```python
from build123d import *

# Parameters (mm, degrees)
BOSS_EXTRU_1_DEPTH      = 10
COQUE1_T                = 2
CONG_1_R                = 4
ENL_V_MAT_EXTRU_1_DEPTH = 10


with BuildPart() as part:
    # Esquisse1 → Boss.-Extru.1 (new body)
    with BuildSketch(Plane.XY):
        with BuildLine():
            Line((-33.546223224, -67.598576794), (32.573776776, -67.598576794))
            ThreePointArc((32.573776776, -67.598576794), (34.341543729, -66.866343747), (35.073776776, -65.098576794))
            Line((35.073776776, -65.098576794), (35.073776776, 67.061423206))
            ThreePointArc((35.073776776, 67.061423206), (34.341543729, 68.829190159), (32.573776776, 69.561423206))
            Line((32.573776776, 69.561423206), (-33.546223224, 69.561423206))
            ThreePointArc((-33.546223224, 69.561423206), (-35.313990177, 68.829190159), (-36.046223224, 67.061423206))
            Line((-36.046223224, 67.061423206), (-36.046223224, -65.098576794))
            ThreePointArc((-36.046223224, -65.098576794), (-35.313990177, -66.866343747), (-33.546223224, -67.598576794))
        make_face()
    extrude(amount=BOSS_EXTRU_1_DEPTH)

    # Coque1
    coque1_openings = [part.faces().sort_by_distance(p)[0] for p in [
        (-0.486223224, 0.981423206, 10),
    ]]
    offset(amount=COQUE1_T, openings=coque1_openings, kind=Kind.INTERSECTION)

    # Congé1
    # the kernel refuses this fillet: 4 mm, written as the material it takes off along each edge
    with BuildSketch(Plane(origin=(32.573776776, 71.561423206, -2), x_dir=(0, 0, 1), z_dir=(-1, 0, 0)), Plane(origin=(-33.546223224, -69.598576794, -2), x_dir=(0, 0, 1), z_dir=(1, 0, 0))) as cong_1_piece_1:
        with BuildLine():
            CenterArc((CONG_1_R, -CONG_1_R), CONG_1_R, 90, 90)
            Line((0, -CONG_1_R), (0, 0))
            Line((0, 0), (CONG_1_R, 0))
        make_face()
    extrude(amount=66.12, mode=Mode.SUBTRACT)
    with BuildSketch(Plane(origin=(32.573776776, 67.061423206, -2), x_dir=(0, 1, 0), z_dir=(-1, 0, 0))) as cong_1_piece_2:
        with BuildLine():
            CenterArc((4.5 - CONG_1_R, -CONG_1_R), CONG_1_R, 0, 90)
            Line((4.5 - CONG_1_R, 0), (4.5, 0))
            Line((4.5, 0), (4.5, -CONG_1_R))
        make_face()
    revolve(axis=Axis((32.573776776, 67.061423206, -2), (0, 0, -1)), revolution_arc=90, mode=Mode.SUBTRACT)
    with BuildSketch(Plane(origin=(37.073776776, -65.098576794, -2), x_dir=(0, 0, 1), z_dir=(0, 1, 0)), Plane(origin=(-38.046223224, 67.061423206, -2), x_dir=(0, 0, 1), z_dir=(0, -1, 0))) as cong_1_piece_3:
        with BuildLine():
            CenterArc((CONG_1_R, -CONG_1_R), CONG_1_R, 90, 90)
            Line((0, -CONG_1_R), (0, 0))
            Line((0, 0), (CONG_1_R, 0))
        make_face()
    extrude(amount=132.16, mode=Mode.SUBTRACT)
    with BuildSketch(Plane(origin=(32.573776776, -65.098576794, -2), x_dir=(1, 0, 0), z_dir=(0, 1, 0))) as cong_1_piece_4:
        with BuildLine():
            CenterArc((4.5 - CONG_1_R, -CONG_1_R), CONG_1_R, 0, 90)
            Line((4.5 - CONG_1_R, 0), (4.5, 0))
            Line((4.5, 0), (4.5, -CONG_1_R))
        make_face()
    revolve(axis=Axis((32.573776776, -65.098576794, -2), (0, 0, -1)), revolution_arc=90, mode=Mode.SUBTRACT)
    with BuildSketch(Plane(origin=(-33.546223224, -65.098576794, -2), x_dir=(0, -1, 0), z_dir=(1, 0, 0))) as cong_1_piece_5:
        with BuildLine():
            CenterArc((4.5 - CONG_1_R, -CONG_1_R), CONG_1_R, 0, 90)
            Line((4.5 - CONG_1_R, 0), (4.5, 0))
            Line((4.5, 0), (4.5, -CONG_1_R))
        make_face()
    revolve(axis=Axis((-33.546223224, -65.098576794, -2), (0, 0, -1)), revolution_arc=90, mode=Mode.SUBTRACT)
    with BuildSketch(Plane(origin=(-33.546223224, 67.061423206, -2), x_dir=(-1, 0, 0), z_dir=(0, -1, 0))) as cong_1_piece_6:
        with BuildLine():
            CenterArc((4.5 - CONG_1_R, -CONG_1_R), CONG_1_R, 0, 90)
            Line((4.5 - CONG_1_R, 0), (4.5, 0))
            Line((4.5, 0), (4.5, -CONG_1_R))
        make_face()
    revolve(axis=Axis((-33.546223224, 67.061423206, -2), (0, 0, -1)), revolution_arc=90, mode=Mode.SUBTRACT)

    # Esquisse2 → Enlèv. mat.-Extru.1 (cut)
    with BuildSketch(Plane(origin=(0, 0, -2), x_dir=(-1, 0, 0), z_dir=(0, 0, -1))):
        with BuildLine():
            Line((-22.841530632, -59.197056867), (23.81397708, -59.197056867))
            ThreePointArc((23.81397708, -59.197056867), (26.642404205, -58.025483992), (27.81397708, -55.197056867))
            Line((27.81397708, -55.197056867), (27.81397708, 57.159903279))
            ThreePointArc((27.81397708, 57.159903279), (26.642404205, 59.988330404), (23.81397708, 61.159903279))
            Line((23.81397708, 61.159903279), (-22.841530632, 61.159903279))
            ThreePointArc((-22.841530632, 61.159903279), (-25.669957756, 59.988330404), (-26.841530632, 57.159903279))
            Line((-26.841530632, 57.159903279), (-26.841530632, -55.197056867))
            ThreePointArc((-26.841530632, -55.197056867), (-25.669957756, -58.025483992), (-22.841530632, -59.197056867))
        make_face()
    extrude(amount=-ENL_V_MAT_EXTRU_1_DEPTH, mode=Mode.SUBTRACT)


solid = part.part
```
The model under review builds one solid part; all positions refer to its coordinate system, in mm. A direction names the side the tool comes from. Round coordinates to 2 decimals unless told otherwise and drop trailing zeros. Order: outer loops, then holes, each group sorted by start corner. A loop starts at its lowest first (then second) coordinate and runs counter-clockwise, first axis right, second up. Notation, with made-up numbers: (-3.5, 87.25) - (26.5, 87.25) arc R17 cw to (26.5, 99.25) - close; hole circle Ø5 at (40, 69.5). An arc over 180 degrees is marked (long way). Answer in a Markdown table with one row per item.
(1) Take a section at A-A on x = -2. Write out the cut boundary in (y, z).
Result set:
| item | result |
|---|---|
| outline | (-69.6, 2) arc R4 ccw to (-65.6, -2) - (-59.2, -2) - (-59.2, 0) - (-67.6, 0) - (-67.6, 10) - (-69.6, 10) - close; (61.16, -2) - (67.56, -2) arc R4 ccw to (71.56, 2) - (71.56, 10) - (69.56, 10) - (69.56, 0) - (61.16, 0) - close |
(2) Take a section at D-D on x = 29. Write out the cut boundary in (y, z).
Result set:
| item | result |
|---|---|
| outline | (-69.6, 2) arc R4 ccw to (-65.6, -2) - (67.56, -2) arc R4 ccw to (71.56, 2) - (71.56, 10) - (69.56, 10) - (69.56, 0) - (-67.6, 0) - (-67.6, 10) - (-69.6, 10) - close |
(3) Mouldability with a two-part tool opening along X and no side actions: class faces 4 (the face through (-1, -67.599, 5)), 5 (the face through (-36.76, -68.25, 5.94)), 6 (the face through (-0.02, 70.42, -0.8)) as released by +X, released by -X, zero draft, split by the parting line, or undercut.
Result set:
| item | result |
|---|---|
| face 4 | undercut |
| face 5 | released by -X |
| face 6 | zero draft |
(4) Clearance check with flat-ended pins moving along their axes: P1, Ø0.6, axis at x = -2, z = -1.5, coming from the +Y side; P2, Ø1, axis at y = 18, z = -1.5, coming from the -X side; P3, Ø1.6, axis at y = 16, z = -1.5, coming from the +X side. State where each tip first meets the part, or that it passes through.
Result set:
| item | result |
|---|---|
| P1 | stops at y = 69.96 |
| P2 | stops at x = -36.69 |
| P3 | stops at x = 36.03 |
(5) Take a section at B-B on y = -15. Write out the cut boundary in (x, z), plus the area to 3 significant figures.
Result set:
| item | result |
|---|---|
| outline | (-38.05, 2) arc R4 ccw to (-34.05, -2) - (-27.81, -2) - (-27.81, 0) - (-36.05, 0) - (-36.05, 10) - (-38.05, 10) - close; (26.84, -2) - (33.07, -2) arc R4 ccw to (37.07, 2) - (37.07, 10) - (35.07, 10) - (35.07, 0) - (26.84, 0) - close |
| area | 74.1 mm2 |
(6) For line 1 (Y direction, x = -9, z = 7.5); line 2 (X direction, y = 63.5, z = 5); line 3 (X direction, y = -35, z = -1.25), list the stretches that pass through material, from the lowest coordinate up. Write a range as from..to.
Result set:
| item | result |
|---|---|
| line 1 | y = -69.6..-67.6, 69.56..71.56 |
| line 2 | x = -38.05..-36.05, 35.07..37.07 |
| line 3 | x = -36.38..-27.81, 26.84..35.41 |
(7) Machinability: for faces 1 (the face through (-30, -4, 0)), 2 (the face through (25.701, -57.994, -1.014)), 3 (the face through (0, 71.561, 6)), which of the approach directions +Z, -Z, +X, -X, +Y, -Y give a long, thin tool a straight path to every point of the face, cutting with its end or side? Answer none if there is none.
Result set:
| item | result |
|---|---|
| face 1 | +Z |
| face 2 | +Z, -Z |
| face 3 | +Z, -Z, +X, -X, +Y |
(8) Take a section at C-C on z = 7.25. Write out the cut boundary in (x, y), plus the area to 3 significant figures.
Result set:
| item | result |
|---|---|
| outline | (-38.05, -65.1) arc R4.5 ccw to (-33.55, -69.6) - (32.57, -69.6) arc R4.5 ccw to (37.07, -65.1) - (37.07, 67.06) arc R4.5 ccw to (32.57, 71.56) - (-33.55, 71.56) arc R4.5 ccw to (-38.05, 67.06) - close; hole (-36.05, -65.1) arc R2.5 ccw to (-33.55, -67.6) - (32.57, -67.6) arc R2.5 ccw to (35.07, -65.1) - (35.07, 67.06) arc R2.5 ccw to (32.57, 69.56) - (-33.55, 69.56) arc R2.5 ccw to (-36.05, 67.06) - close |
| area | 837 mm2 |
